Model file for the job. Use its own axes, mm. A direction names the side the tool comes from. Coordinates: 2 decimals unless noted, no trailing zeros. Write each loop counter-clockwise with the first axis right and the second up, starting at its lowest first coordinate (ties: lowest second). Pieces come first, ordered by that corner, then holes. Notation, with made-up numbers: M 67.25,52.5 L 93.25,52.5 A28 ccw 93.25,91.5 Z; hole C 88.25,77.25 d5. An arc over 180 degrees is marked long. One line per question, with ' | ' between items. Start each with the question number.
(1) Cut at A-A (z = 2.25). Write the cut outline in (x, y).
(2) Tool access for faces 1 (the face through (3, 36, 0)), 2 (the face through (4.68, 69.23, 1.48)), 3 (the face through (1.25, 34, 1)), 4 (the face through (5.25, 33, 1)), 5 (the face through (6.5, 67.2, 1.5)): list every direction of +Z, -Z, +X, -X, +Y, -Y with a clear straight run to the whole face (end or side of a thin tool).
(3) Wall check: probe 1 along Y at (x, z) = (3.25, 1.2); probe 2 along X at (y, z) = (18, 2.25); probe 3 along Z at (x, y) = (1.5, 47). Give the ranges that are in metal, low to high.
(4) Two-plate mould, pull along Y, no slides. Class faces 6 (the face through (3, 36, 3)), 7 (the face through (3.312, 65.425, 1.479)), 8 (the face through (1.827, 69.217, 1.479)), 9 (the face through (4.636, 2.35, 7.93)): +Y half, -Y half, draft (parallel to the pull), parting line (faces both ways), or undercut.
(5) Cut at B-B (y = 42). Write the cut outline in (x, z), plus the area to 3 significant figures.
(6) Flat gauge pins, fed straight in: pin 1 Ø2.5 at (y, z) = (25.5, 2) entering from -X; pin 2 Ø2 at (x, y) = (4, 29.5) entering from +Z; pin 3 Ø1.5 at (x, z) = (3, 9) entering from +Y. Where does each tip first touch, or does it go through?
from build123d import *

# Parameters (mm, degrees)
F1_DEPTH = 3
F2_R     = 1.5
F3_DEPTH = 10


# Not quite as in the source:
# - a feature names something its author has since deleted; it is built from what else it names


with BuildPart() as f1:
    # F0 (on Top) → F1 (new body)
    with BuildSketch(Plane.XY):
        with BuildLine():
            ThreePointArc((3.25, 63.9241337907), (2.1924432633, 64.1010126169), (1.25, 64.6123960992))
            Line((1.25, 64.6123960992), (1.25, 2.9241337907))
            ThreePointArc((1.25, 2.9241337907), (1.8357864376, 4.338347353), (3.25, 4.9241337907))
            Line((3.25, 4.9241337907), (3.25, 63.9241337907))
        make_face()
        with BuildLine():
            ThreePointArc((3.25, 4.9241337907), (1.8357864376, 4.338347353), (1.25, 2.9241337907))
            ThreePointArc((1.25, 2.9241337907), (1.8357864376, 1.5099202283), (3.25, 0.9241337907))
            Line((3.25, 0.9241337907), (3.25, 4.9241337907))
        make_face()
        with BuildLine():
            ThreePointArc((5.25, 64.6123960992), (4.3075567367, 64.1010126169), (3.25, 63.9241337907))
            Line((3.25, 63.9241337907), (3.25, 4.9241337907))
            ThreePointArc((3.25, 4.9241337907), (4.6642135624, 4.338347353), (5.25, 2.9241337907))
            Line((5.25, 2.9241337907), (5.25, 64.6123960992))
        make_face()
        with BuildLine():
            ThreePointArc((5.25, 2.9241337907), (4.6642135624, 4.338347353), (3.25, 4.9241337907))
            Line((3.25, 4.9241337907), (3.25, 0.9241337907))
            ThreePointArc((3.25, 0.9241337907), (4.6642135624, 1.5099202283), (5.25, 2.9241337907))
        make_face()
        with BuildLine():
            Line((2.25, 68.6102744523), (1.3928571429, 69.8412521623))
            ThreePointArc((1.3928571429, 69.8412521623), (0.0012122742, 67.2628936507), (1.25, 64.6123960992))
            ThreePointArc((1.25, 64.6123960992), (2.1924432633, 64.1010126169), (3.25, 63.9241337907))
            ThreePointArc((3.25, 63.9241337907), (4.3075567367, 64.1010126169), (5.25, 64.6123960992))
            ThreePointArc((5.25, 64.6123960992), (6.4987877258, 67.2628936507), (5.1071428571, 69.8412521623))
            Line((5.1071428571, 69.8412521623), (4.25, 68.6102744523))
            ThreePointArc((4.25, 68.6102744523), (3.25, 65.4241337907), (2.25, 68.6102744523))
        make_face()
    extrude(amount=F1_DEPTH)

    # F2 (on face) → F3 (join)
    with BuildSketch(Plane.XY.offset(3)):
        with Locations((3.25, 2.9241337907)):
            Circle(F2_R)
    extrude(amount=F3_DEPTH)


solid = f1.part
Filled in:
1) outline: M 1.25,2.92 A2 ccw 5.25,2.92 L 5.25,64.61 A3.25 ccw 5.11,69.84 L 4.25,68.61 A1.75 cw long 2.25,68.61 L 1.39,69.84 A3.25 ccw 1.25,64.61 Z
2) face 1: -Z, +X, -X, +Y, -Y | face 2: +Z, -Z, +Y | face 3: +Z, -Z, -X, -Y | face 4: +Z, -Z, +X, -Y | face 5: +Z, -Z, +X
3) probe 1: 0.92 to 65.42 | probe 2: 1.25 to 5.25 | probe 3: 0 to 3
4) face 6: draft | face 7: undercut | face 8: +Y half | face 9: parting line
5) outline: M 1.25,0 L 5.25,0 L 5.25,3 L 1.25,3 Z | area: 12.0 mm²
6) pin 1: x = 1.25 | pin 2: z = 3 | pin 3: y = 4.42
